```python
from build123d import *

# Parameters (mm, degrees)
SKETCH_1_W                   = 18.5
SKETCH_1_H                   = 4
HOLE_WIZARD_M3_1_D           = 3.5
HOLE_WIZARD_M3_1_CBORE_D     = 5.5
HOLE_WIZARD_M3_1_CBORE_DEPTH = 2
SKETCH_9_R                   = 4.078764036
EXTRUDE_2_DEPTH              = 4
SKETCH_10_R                  = 3
EXTRUDE_3_DEPTH              = 8
CUT_EXTRUDE_START            = -6.5
CUT_EXTRUDE_2_DEPTH          = 6.5
PATTERN_CIRCULAR_1_COUNT     = 3
PATTERN_CIRCULAR_1_ANGLE     = 120
SKETCH_13_W                  = 2.125984269
SKETCH_13_H                  = 7.532431529
EXTRUDE_4_DEPTH              = 0.8


with BuildPart() as part:
    # Sketch 1 → Revolve 1 (revolve)
    with BuildSketch(Plane.XY.offset(0.922906258), mode=Mode.PRIVATE) as revolve_1_sk:
        with Locations((9.859359688, 2)):
            Rectangle(SKETCH_1_W, SKETCH_1_H)
    revolve(revolve_1_sk.sketch.rotate(Axis((0.609359688, 4, 0.922906258), (0, -1, 0)), 270), axis=Axis((0.609359688, 4, 0.922906258), (0, -1, 0)))

    # Hole Wizard M3 _1 (through all)
    with Locations(Plane(origin=(0, 4, 0), x_dir=(1, 0, 0), z_dir=(0, 1, 0))):
        with Locations((-11.081983263, -7.672906258), (12.300702639, -7.672906258), (0.609359688, 12.577093742)):
            hole_wizard_m3_1 = CounterBoreHole(HOLE_WIZARD_M3_1_D / 2, HOLE_WIZARD_M3_1_CBORE_D / 2, HOLE_WIZARD_M3_1_CBORE_DEPTH)

    # Sketch 9 → Extrude 2 (add)
    with BuildSketch(Plane.XZ):
        with Locations((0.609359688, 0.922906258)):
            Circle(SKETCH_9_R)
    extrude(amount=-EXTRUDE_2_DEPTH)

    # Sketch 10 → Extrude 3 (add)
    with BuildSketch(Plane(origin=(0, 4, 0), x_dir=(1, 0, 0), z_dir=(0, 1, 0))):
        with Locations(Location((0.609359688, -0.922906258, 0), (0, 0, 270))):
            Circle(SKETCH_10_R)
    extrude(amount=EXTRUDE_3_DEPTH)

    # Sketch 11 → Cut-Extrude 2 (cut)
    with BuildSketch(Plane(origin=(0, 12, 0), x_dir=(1, 0, 0), z_dir=(0, 1, 0)).offset(CUT_EXTRUDE_START)):
        with BuildLine():
            Line((2.905866026, 1.007393885), (2.905866026, -2.853206401))
            ThreePointArc((2.905866026, -2.853206401), (3.609359688, -0.922906258), (2.905866026, 1.007393885))
        make_face()
    extrude(amount=CUT_EXTRUDE_2_DEPTH, mode=Mode.SUBTRACT)

    # Pattern Circular 1: Hole Wizard M3 _1 ×3 about axis
    pattern_circular_1_axis = Axis((0.609359688, 0, 0.922906258), (0, -1, 0))
    for i in range(1, PATTERN_CIRCULAR_1_COUNT):
        add(hole_wizard_m3_1.rotate(pattern_circular_1_axis, i * PATTERN_CIRCULAR_1_ANGLE / (PATTERN_CIRCULAR_1_COUNT - 1)), mode=Mode.SUBTRACT)


with BuildPart() as body_2:
    # Move Body 3: copy of part
    add(part.part.moved(Location((0, 0, 43.295994543))))


with BuildPart() as part_1:
    add(part.part)

    add(body_2.part)  # Extrude 4 merges body 2
    # Sketch 13 → Extrude 4 (add)
    with BuildSketch(Plane.XZ):
        with Locations((-0.453632447, 22.075248032)):
            Rectangle(SKETCH_13_W, SKETCH_13_H)
    extrude(amount=-EXTRUDE_4_DEPTH)


solid = part_1.part
```
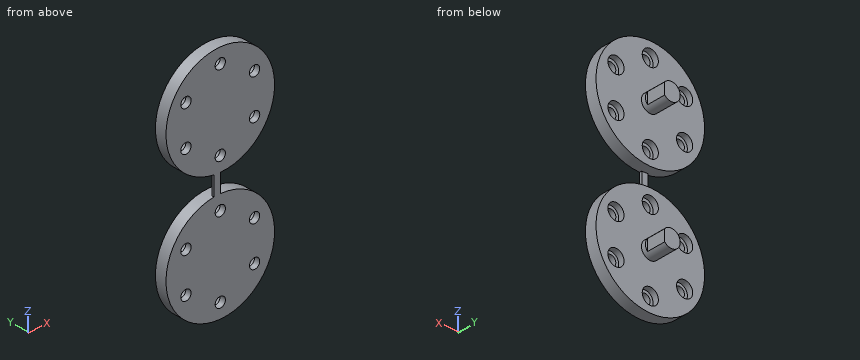
Geometry check sheet. Reference: the model listing, model coordinates, mm. Give positions to 0.01 mm unless a question says otherwise; leave off trailing zeros. Loops run counter-clockwise (first coordinate to the right, second up) from the corner with the lowest first, then second, coordinate; pieces in that order, holes last. Notation, with made-up numbers: (81, -9.75) - (98, -9.75) arc R22 cw to (98, 27.25) - close; hole circle Ø11 at (-18, 33.5). An arc over 180 degrees is marked (long way). Use CSV: the item, a comma, the result in double quotes. Start each with the question number.
Q1. Scan lines: probe 1 along Y at (x, z) = (-3, -3); probe 2 along X at (y, z) = (2.75, 33); probe 3 along Z at (x, y) = (-2, 9). Record each from-to range of solid material in increasing order. Write a range as from..to.
Q2. Go/stop test with flat-tipped pins: pin 1 Ø9 at (x, z) = (-11.08, 37.47) entering from -Y; pin 2 Ø7 at (x, z) = (-11.08, 7.67) entering from +Y; pin 3 Ø3 at (y, z) = (9.5, 0.5) entering from +X; pin 4 Ø1.5 at (x, y) = (-10, 2.5) entering from +Z. Record where each tip stops, or that it passes through.
Q3. Section check B-B, the plane z = 50. Record the cut outline in (x, y).
Q4. Section check D-D, the plane z = 24. Record the cut outline in (x, y).
Q5. Section check C-C, the plane x = -6. Record the cut outline in (y, z).
Q6. Section check A-A, the plane y = 3. Count the separate pieces of the cut face and the enclosed holes in it, and give its area (3 significant figures).
Findings below:
1,probe 1,"y = 0..4"
1,probe 2,"x = -14.1..-0.93, 2.15..15.32"
1,probe 3,"z = -0.56..2.4, 42.74..45.7"
2,pin 1,"stops at y = 0"
2,pin 2,"stops at y = 4"
2,pin 3,"stops at x = 2.91"
2,pin 4,"stops at z = 59.87"
3,outline,"(-16.96, 0) - (-12.54, 0) - (-12.54, 2) - (-13.66, 2) - (-13.66, 4) - (-16.96, 4) - close; (-9.62, 0) - (10.84, 0) - (10.84, 2) - (9.73, 2) - (9.73, 4) - (-8.51, 4) - (-8.51, 2) - (-9.62, 2) - close; (13.76, 0) - (18.18, 0) - (18.18, 4) - (14.87, 4) - (14.87, 2) - (13.76, 2) - close"
4,outline,"(-1.52, 0) - (0.61, 0) - (0.61, 0.8) - (-1.52, 0.8) - close"
5,outline,"(0, -16.36) - (4, -16.36) - (4, 18.2) - (0, 18.2) - close; (0, 26.94) - (4, 26.94) - (4, 61.5) - (0, 61.5) - close"
6,separate pieces,"2"
6,enclosed holes,"12"
6,area,"1,870 mm^2"
